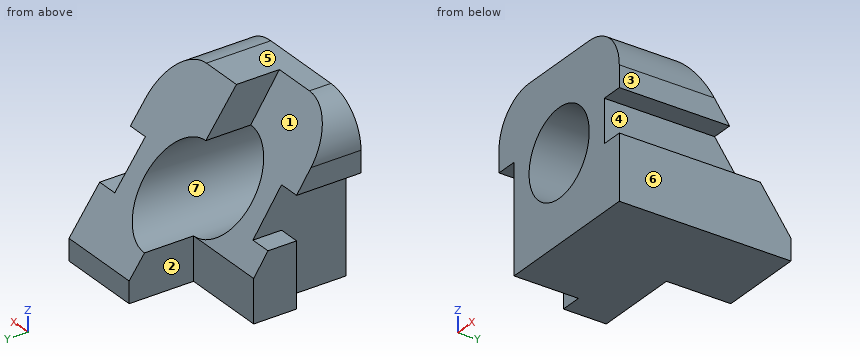
from build123d import *

# Parameters (mm, degrees)
SKETCH1_W           = 40
SKETCH1_H           = 40
BOSS_EXTRUDE1_DEPTH = 40
SKETCH2_R           = 10
CUT_EXTRUDE1_DEPTH  = 41
SKETCH3_W           = 5
SKETCH3_H           = 10
CUT_EXTRUDE2_DEPTH  = 41
CUT_EXTRUDE5_DEPTH  = 41
CUT_EXTRUDE6_DEPTH  = 41
SKETCH8_W           = 15
SKETCH8_H           = 15
CUT_EXTRUDE7_DEPTH  = 5
SKETCH9_W           = 15
SKETCH9_H           = 15
CUT_EXTRUDE8_DEPTH  = 20
CUT_EXTRUDE9_DEPTH  = 20
CUT_EXTRUDE10_DEPTH = 20


with BuildPart() as part:
    # Sketch1 → Boss-Extrude1 (new body)
    with BuildSketch(Plane.XY):
        Rectangle(SKETCH1_W, SKETCH1_H)
    extrude(amount=BOSS_EXTRUDE1_DEPTH)

    # Sketch2 → Cut-Extrude1 (cut, through all)
    with BuildSketch(Plane(origin=(0, 20, 0), x_dir=(1, 0, 0), z_dir=(0, 1, 0))):
        with Locations((0, -20)):
            Circle(SKETCH2_R)
    extrude(amount=-CUT_EXTRUDE1_DEPTH, mode=Mode.SUBTRACT)

    # Sketch3 → Cut-Extrude2 (cut, through all)
    with BuildSketch(Plane(origin=(0, 20, 0), x_dir=(1, 0, 0), z_dir=(0, 1, 0))):
        with Locations((17.5, -20)):
            Rectangle(SKETCH3_W, SKETCH3_H)
        with Locations((-17.5, -20)):
            Rectangle(SKETCH3_W, SKETCH3_H)
    extrude(amount=-CUT_EXTRUDE2_DEPTH, mode=Mode.SUBTRACT)

    # Sketch5 → Cut-Extrude5 (cut, through all)
    with BuildSketch(Plane(origin=(0, 20, 0), x_dir=(1, 0, 0), z_dir=(0, 1, 0))):
        with BuildLine():
            Line((-10, -40), (-20, -40))
            Line((-20, -40), (-20, -30))
            ThreePointArc((-20, -30), (-17.071067812, -37.071067812), (-10, -40))
        make_face()
    extrude(amount=-CUT_EXTRUDE5_DEPTH, mode=Mode.SUBTRACT)

    # Sketch7 → Cut-Extrude6 (cut, through all)
    with BuildSketch(Plane(origin=(0, 20, 0), x_dir=(1, 0, 0), z_dir=(0, 1, 0))):
        with BuildLine():
            Line((20, -30), (20, -40))
            Line((20, -40), (10, -40))
            ThreePointArc((10, -40), (17.071067812, -37.071067812), (20, -30))
        make_face()
    extrude(amount=-CUT_EXTRUDE6_DEPTH, mode=Mode.SUBTRACT)

    # Sketch8 → Cut-Extrude7 (cut)
    with BuildSketch(Plane.ZY.offset(20)):
        with Locations((7.5, -12.5)):
            Rectangle(SKETCH8_W, SKETCH8_H)
    extrude(amount=-CUT_EXTRUDE7_DEPTH, mode=Mode.SUBTRACT)

    # Sketch9 → Cut-Extrude8 (cut)
    with BuildSketch(Plane.ZY.offset(20)):
        with Locations((7.5, 12.5)):
            Rectangle(SKETCH9_W, SKETCH9_H)
    extrude(amount=-CUT_EXTRUDE8_DEPTH, mode=Mode.SUBTRACT)

    # Sketch10 → Cut-Extrude9 (cut)
    with BuildSketch(Plane(origin=(-20, 0, 0), x_dir=(0, 0, -1), z_dir=(1, 0, 0))):
        Polygon((-10, 5), (-40, -15), (-40, 20), (-10, 20), align=None)
    extrude(amount=CUT_EXTRUDE9_DEPTH, mode=Mode.SUBTRACT)

    # Sketch11 → Cut-Extrude10 (cut)
    with BuildSketch(Plane(origin=(20, 0, 0), x_dir=(0, 0, -1), z_dir=(1, 0, 0))):
        Polygon((-5, 20), (-40, -5), (-40, 20), align=None)
    extrude(amount=-CUT_EXTRUDE10_DEPTH, mode=Mode.SUBTRACT)


solid = part.part
Geometry: final body of the model. Coordinates: model frame, mm. Face numbers are marked on the shaded views. A direction names the side the tool comes from. Give positions to 0.01 mm unless a question says otherwise; leave off trailing zeros. Order: outer loops, then holes, each group sorted by start corner. A loop starts at its lowest first (then second) coordinate and runs counter-clockwise, first axis right, second up. Notation, with made-up numbers: (34, 20) -> (43, 20) arc R32 ccw to (43, 48) -> close; hole circle Ø10 at (86, -36). An arc over 180 degrees is marked (long way). Put each result on its own line as item: value.
Q1. Section A-A, the plane x = 1.5. Return loops of the section in (y, z).
Here are the results:
outline: (-20, 0) -> (20, 0) -> (20, 5) -> (16.35, 10.11) -> (-20, 10.11) -> close; (-20, 29.89) -> (2.22, 29.89) -> (-5, 40) -> (-20, 40) -> close
Q2. Reachability of the marked faces 1, 2 and 3 from +Z, -Z, +X, -X, +Y, -Y: full face, straight path, thin tool, end or side. Return the list, or none.
Here are the results:
face 1: +Z, -X, +Y
face 2: +Z, -Z, -X, +Y
face 3: +Z, -Z, +X, +Y, -Y
Q3. Material intervals for L1, parallel to X at y = -4, z = 20; L2, parallel to Y at x = 14, z = 30; L3, parallel to Y at x = 13, z = 25, sorted ascending.
Here are the results:
L1: x = -15 to -10, 10 to 15
L2: y = -20 to 2.14
L3: y = -20 to 5.71
Q4. Pin query (flat end, axial travel): pin 1 (8 mm diameter, centred on x = -7.5, z = 35, fed in from +Y); pin 2 (3 mm diameter, centred on x = -14.5, z = 3.5, fed in from +Y); pin 3 (12 mm diameter, centred on x = 0.5, z = 30.5, fed in from +Y); pin 4 (11 mm diameter, centred on y = -3.5, z = 20, fed in from +X). Return the tip coordinate at first contact, or that it passes through.
Here are the results:
pin 1: stops at y = -9
pin 2: stops at y = 5
pin 3: stops at y = 3.55
pin 4: stops at x = 20
Q5. Section C-C, the plane z = 12.5. Return loops of the section in (x, y).
Here are the results:
outline: (-20, -5) -> (-15, -5) -> (-15, -20) -> (-6.61, -20) -> (-6.61, 3.33) -> (-20, 3.33) -> close; (6.61, -20) -> (20, -20) -> (20, 14.64) -> (6.61, 14.64) -> close
Q6. Section B-B, the plane y = -16.5. Return loops of the section in (x, z), then the cut area to 3 significant figures.
Here are the results:
outline: (-20, 25) -> (-15, 25) -> (-15, 0) -> (20, 0) -> (20, 15) -> (15, 15) -> (15, 25) -> (20, 25) -> (20, 30) arc R10 ccw to (10, 40) -> (-10, 40) arc R10 ccw to (-20, 30) -> close; hole circle Ø20 at (0, 20)
area: 1,070 mm^2
Q7. Section D-D, the plane y = -6. Return loops of the section in (x, z), then the cut area to 3 significant figures.
Here are the results:
outline: (-20, 25) -> (-15, 25) -> (-15, 0) -> (20, 0) -> (20, 15) -> (15, 15) -> (15, 25) -> (20, 25) -> (20, 30) arc R10 ccw to (10, 40) -> (0, 40) -> (0, 30) arc R10 cw (long way) to (-7.6, 26.5) -> (-20, 26.5) -> close
area: 838 mm^2
Q8. Draft query along Z for the marked faces 4, 5, 6 and 7. Return one class per face: released by +Z, released by -Z, zero draft, split by the parting line, or undercut.
Here are the results:
face 4: undercut
face 5: released by +Z
face 6: zero draft
face 7: undercut
